```python
from build123d import *

# Parameters (mm, degrees)
F1_DEPTH = 914.4


with BuildPart() as f1:
    # F0 (on Front) → F1 (new body)
    with BuildSketch(Plane.XZ):
        with BuildLine():
            Line((-114.3483273342, -1.1068779329), (-127, 0))
            ThreePointArc((-127, 0), (-124.8046262141, -23.5118114054), (-118.2944051093, -46.2107532923))
            Line((-118.2944051093, -46.2107532923), (-114.3483273342, -1.1068779329))
        make_face()
        with BuildLine():
            ThreePointArc((-118.2944051093, -46.2107532923), (-124.8046262141, -23.5118114054), (-127, 0))
            Line((-127, 0), (-135.8550234632, -101.2133813261))
            Line((-135.8550234632, -101.2133813261), (-76.7127853785, -101.2133813261))
            ThreePointArc((-76.7127853785, -101.2133813261), (-84.1331171102, -95.134739214), (-91.0734940925, -88.5133813261))
            Line((-91.0734940925, -88.5133813261), (-121.9954054996, -88.5133813261))
            Line((-121.9954054996, -88.5133813261), (-118.2944051093, -46.2107532923))
        make_face()
        with BuildLine():
            ThreePointArc((76.7127853785, -101.2133813261), (84.1331171102, -95.134739214), (91.0734940925, -88.5133813261))
            Line((91.0734940925, -88.5133813261), (0, -88.5133813261))
            Line((0, -88.5133813261), (-91.0734940925, -88.5133813261))
            ThreePointArc((-91.0734940925, -88.5133813261), (-84.1331171102, -95.134739214), (-76.7127853785, -101.2133813261))
            Line((-76.7127853785, -101.2133813261), (0, -101.2133813261))
            Line((0, -101.2133813261), (76.7127853785, -101.2133813261))
        make_face()
        with BuildLine():
            Line((135.8550234632, -101.2133813261), (127, 0))
            ThreePointArc((127, 0), (124.8046262141, -23.5118114054), (118.2944051093, -46.2107532923))
            Line((118.2944051093, -46.2107532923), (121.9954054996, -88.5133813261))
            Line((121.9954054996, -88.5133813261), (91.0734940925, -88.5133813261))
            ThreePointArc((91.0734940925, -88.5133813261), (84.1331171102, -95.134739214), (76.7127853785, -101.2133813261))
            Line((76.7127853785, -101.2133813261), (135.8550234632, -101.2133813261))
        make_face()
        with BuildLine():
            ThreePointArc((118.2944051093, -46.2107532923), (124.8046262141, -23.5118114054), (127, 0))
            Line((127, 0), (114.3483273342, -1.1068779329))
            Line((114.3483273342, -1.1068779329), (118.2944051093, -46.2107532923))
        make_face()
    extrude(amount=F1_DEPTH)


solid = f1.part
```
Check sheet for the modelled part. Datum: model origin and axes. Units: mm. Round coordinates to 2 decimals unless told otherwise and drop trailing zeros. Loops run counter-clockwise (first coordinate to the right, second up) from the corner with the lowest first, then second, coordinate; pieces in that order, holes last. Notation, with made-up numbers: M -24.5,36.25 L 13.5,36.25 A23 ccw 13.5,66.25 Z; hole C 7.25,-10 d1. An arc over 180 degrees is marked long. Answer as a JSON object with one key per item and string values.
1. Section check B-B (y = -735). Record the boundary of the cut face in (x, z), plus the area to 3 significant figures.
Reply:
{"outline": "M -135.86,-101.21 L 135.86,-101.21 L 127,0 L 114.35,-1.11 L 122,-88.51 L -122,-88.51 L -114.35,-1.11 L -127,0 Z", "area": "5,680 mm²"}
2. Mould release check, pull along X, two halves, no side actions. Record for faces 1 (the flat face through (9, 0, -92)), 2 (the flat face through (2, -451, -88.513)), 3 (the flat face through (131.49, -450.8, -51.32)): pulls with the +X half, pulls with the -X half, needs draft (parallel to the pull), parting line crosses it, or undercut.
Reply:
{"face 1": "needs draft", "face 2": "undercut", "face 3": "pulls with the +X half"}
3. Section check A-A (z = -37.5). Record the boundary of the cut face in (x, y), plus the area to 3 significant figures.
Reply:
{"outline": "M -130.28,-914.4 L -117.53,-914.4 L -117.53,0 L -130.28,0 Z; M 117.53,-914.4 L 130.28,-914.4 L 130.28,0 L 117.53,0 Z", "area": "23,300 mm²"}
4. Gauge pin test, flat ends, axial feed: P1, Ø3, axis at y = -317, z = -50.5, coming from the +X side; P2, Ø5, axis at x = -52.5, y = -472.5, coming from the +Z side; P3, Ø8, axis at y = -341, z = -56, coming from the +X side. Record the tip position at first contact, or that the pin passes through.
Reply:
{"P1": "stops at x = 131.55", "P2": "stops at z = -88.51", "P3": "stops at x = 132.25"}
5. Section check C-C (x = 1). Record the boundary of the cut face in (y, z), plus the area to 3 significant figures.
Reply:
{"outline": "M -914.4,-101.21 L 0,-101.21 L 0,-88.51 L -914.4,-88.51 Z", "area": "11,600 mm²"}
6. Scan lines: line 1 (Z direction, x = 35, y = -540); line 2 (X direction, y = -595, z = -13.5); line 3 (X direction, y = -86.5, z = -45). Record each from-to range of solid material in increasing order.
Reply:
{"line 1": "z = -101.21 to -88.51", "line 2": "x = -128.18 to -115.43, 115.43 to 128.18", "line 3": "x = -130.94 to -118.19, 118.19 to 130.94"}
